from build123d import *

# Parameters (mm, degrees)
F0_R     = 6.25
F0_R_2   = 3.25
F1_DEPTH = 10
F2_R     = 5
F2_R_2   = 3.25
F3_DEPTH = 12
F6_R     = 6.25
F7_DEPTH = 2
F8_SIZE  = 1


with BuildPart() as f1:
    # F0 (on Right) → F1 (new body)
    with BuildSketch(Plane.YZ):
        Circle(F0_R)
        Circle(F0_R_2, mode=Mode.SUBTRACT)
    extrude(amount=F1_DEPTH)

    # F2 (on face) → F3 (join)
    with BuildSketch(Plane(origin=(0, 0, 0), x_dir=(0, -1, 0), z_dir=(-1, 0, 0))):
        Circle(F2_R)
        Circle(F2_R_2, mode=Mode.SUBTRACT)
    extrude(amount=F3_DEPTH)

    # F4 (on Front) → F5 (revolve, cut)
    with BuildSketch(Plane.XZ):
        Polygon((-10, 5), (-12, 5), (-12, 4), align=None)
        Polygon((-8, 4), (-6, 5), (-8, 5), align=None)
        Polygon((-4, 4), (-2, 5), (-4, 5), align=None)
    revolve(axis=Axis((-10, 0, 0), (-1, 0, 0)), mode=Mode.SUBTRACT)

    # F6 (on face) → F7 (join)
    with BuildSketch(Plane.YZ.offset(10)):
        Circle(F6_R)
    extrude(amount=-F7_DEPTH)

    # F8
    f8_edges = [f1.edges().sort_by_distance(p)[0] for p in [
        (10, -6.25, 0),
        (0, -6.25, 0),
    ]]
    chamfer(f8_edges, length=F8_SIZE)


solid = f1.part
Design review of the part built by this model. Coordinates are the model's own, in mm. A direction names the side the tool comes from. Round coordinates to 2 decimals unless told otherwise and drop trailing zeros. Write each loop counter-clockwise with the first axis right and the second up, starting at its lowest first coordinate (ties: lowest second). Pieces come first, ordered by that corner, then holes. Notation, with made-up numbers: (82.5, 17) - (99.5, 17) arc R9 ccw to (99.5, 21) - close; hole circle Ø10 at (64.5, 49.25). An arc over 180 degrees is marked (long way). Return JSON: item names as keys, results as strings. Group by question number.
Item 1: Machinability: for faces 1 (the face through (-12, 2, 3)), 2 (the face through (8, 0, 0)), which of the approach directions +Z, -Z, +X, -X, +Y, -Y give a long, thin tool a straight path to every point of the face, cutting with its end or side? Answer none if there is none.
Item 2: We need section A-A on x = -5. Write out the cut boundary in (y, z).
Item 3: Insertion check: P1, Ø4, axis at x = 0, y = 0, coming from the -Z side; P2, Ø3, axis at y = 0.5, z = -0.5, coming from the -X side; P3, Ø2, axis at y = 5, z = -1, coming from the -X side; P4, Ø5, axis at x = -8, y = 1, coming from the +Z side. Each pin has a flat end and moves straight along its axis. Give the tip position at first contact, or say it passes through.
Item 4: For probe 1 along Z at (x, y) = (4.5, 0); probe 2 along Z at (x, y) = (-5.5, 0); probe 3 along X at (y, z) = (-4.25, 3), list the stretches that pass through material, from the lowest coordinate up. Write a range as [from, to].
Item 5: We need section D-D on z = 4.5. Give the number of separate pieces and of enclosed holes in the cut face, and give its area (3 significant figures).
Model answer:
{
 "1": {"face 1": "+Z, -Z, -X, +Y, -Y", "face 2": "-X"},
 "2": {"outline": "circle Ø10 at (0, 0); hole circle Ø6.5 at (0, 0)"},
 "3": {"P1": "stops at z = -6.25", "P2": "stops at x = 8", "P3": "stops at x = -11.8", "P4": "stops at z = 5"},
 "4": {"probe 1": "z = [-6.25, -3.25], [3.25, 6.25]", "probe 2": "z = [-5, -3.25], [3.25, 5]", "probe 3": "x = [0, 10]"},
 "5": {"separate pieces": "3", "enclosed holes": "0", "area": "118 mm²"}
}
